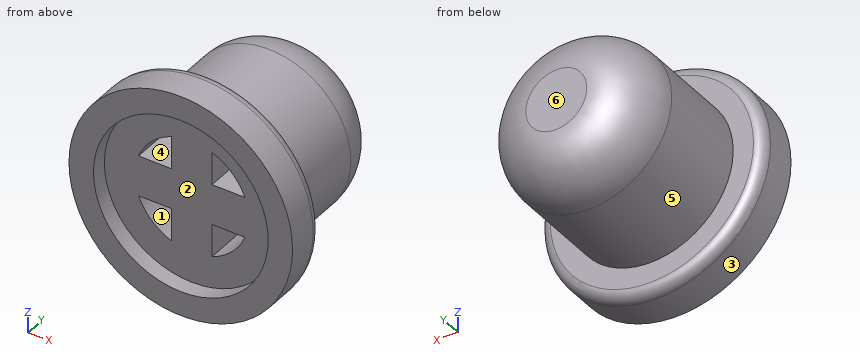
Autodesk Inventor part; units mm, degrees
ref_plane "YZ Plane" through (0, 0, 0) normal (1, 0, 0) x (0, 1, 0)
ref_plane "XZ Plane" through (0, 0, 0) normal (0, 1, 0) x (-1, 0, 0)
ref_plane "XY Plane" through (0, 0, 0) normal (0, 0, 1) x (1, 0, 0)
sketch "Esquisse1" plane through (0, 0, 0) normal (0, 1, 0) x (-1, 0, 0)
  circle A0 centre (0, 0) radius 4
  dimension "d0" = 8
extrude "Extrusion1" add sketch "Esquisse1" along normal blind 7
fillet "Congé1" radius 2.5 1 edges at (4, 7, 0)
sketch "Esquisse2" plane through (0, 0, 0) normal (0, -1, 0) x (1, 0, 0)
  circle A0 centre (0, 0) radius 5.5
  dimension "d4" = 11
extrude "Extrusion2" add sketch "Esquisse2" along normal blind 2
sketch "Esquisse3" plane through (0, -2, 0) normal (0, -1, 0) x (1, 0, 0)
  point P0 (0, 0)
shell "Coque1" thickness 1.2 removed faces 1 at (1.6766, -2, 0.4132)
sketch "Esquisse4" plane through (0, -1.2, 0) normal (0, -1, 0) x (1, 0, 0)
  line L0 (3.5, 1) -> (-3.5, 1)
  line L1 (-3.5, 1) -> (-3.5, -1)
  line L2 (-3.5, -1) -> (3.5, -1)
  line L3 (3.5, -1) -> (3.5, 1)
  line L4 (1, 3.5) -> (-1, 3.5)
  line L5 (-1, 3.5) -> (-1, -3.5)
  line L6 (-1, -3.5) -> (1, -3.5)
  line L7 (1, -3.5) -> (1, 3.5)
  point P0 (0, 0)
  dimension "d8" = 2
  dimension "d9" = 2
  dimension "d10" = 7
  dimension "d11" = 3.5
  dimension "d12" = 7
  dimension "d13" = 3.5
  dimension "d14" = 1
  dimension "d15" = 1
extrude "Extrusion3" add sketch "Esquisse4" against normal blind 2
fillet "Congé2" radius 0.5 1 edges at (-5.5, 0, 0)
equation "\"d9\" = d8"
equation "\"d12\" = d10"
properties part number "Button" material "Plastique ABS"
Source: CAD feature listing. Evaluate the final solid. Frame: model axes, mm. Face numbers are marked on the shaded views. A direction names the side the tool comes from. Coordinates: 2 decimals unless noted, no trailing zeros. Answer in a Markdown table with one row per item.
Q1. Set-up query: the marked faces 4, 5 and 6. Return all of +Z, -Z, +X, -X, +Y, -Y with unobstructed straight access to the full face (end or side cutting, diameter ignored); none if empty.
Answers below:
| item | result |
|---|---|
| face 4 | -Y |
| face 5 | +Y |
| face 6 | +Z, -Z, +X, -X, +Y |
Q2. Draft query along Y for the marked faces 1, 2 and 3. Return one class per face: pulls with the +Y half, pulls with the -Y half, needs draft (parallel to the pull), parting line crosses it, or undercut.
Answers below:
| item | result |
|---|---|
| face 1 | undercut |
| face 2 | pulls with the -Y half |
| face 3 | needs draft |
Q3. First-contact query: pin 1 (0.8 mm diameter, centred on y = 0, z = 1.5, fed in from -X); pin 2 (0.5 mm diameter, centred on y = 0, z = 1.5, fed in from +X); pin 3 (5 mm diameter, centred on y = 4, z = 3, fed in from -X); pin 4 (5 mm diameter, centred on x = -2.5, z = 1, fed in from +Y). Flat tips, straight axial feed; report the tip coordinate or a pass-through.
Answers below:
| item | result |
|---|---|
| pin 1 | stops at x = -5.32 |
| pin 2 | stops at x = 5.24 |
| pin 3 | stops at x = -3.97 |
| pin 4 | stops at y = 7 |
Q4. Ray query, probe 1 along X at (y, z) = (-0.5, -1.25); probe 2 along Y at (x, z) = (-0.5, 0); probe 3 along Z at (x, y) = (0, -1.75). Return the intervals inside material, ascending. Write a range as from..to.
Answers below:
| item | result |
|---|---|
| probe 1 | x = -5.36..-2.51, -1..1, 2.51..5.36 |
| probe 2 | y = -1.2..0.8, 5.8..7 |
| probe 3 | z = -5.5..-4.3, 4.3..5.5 |
